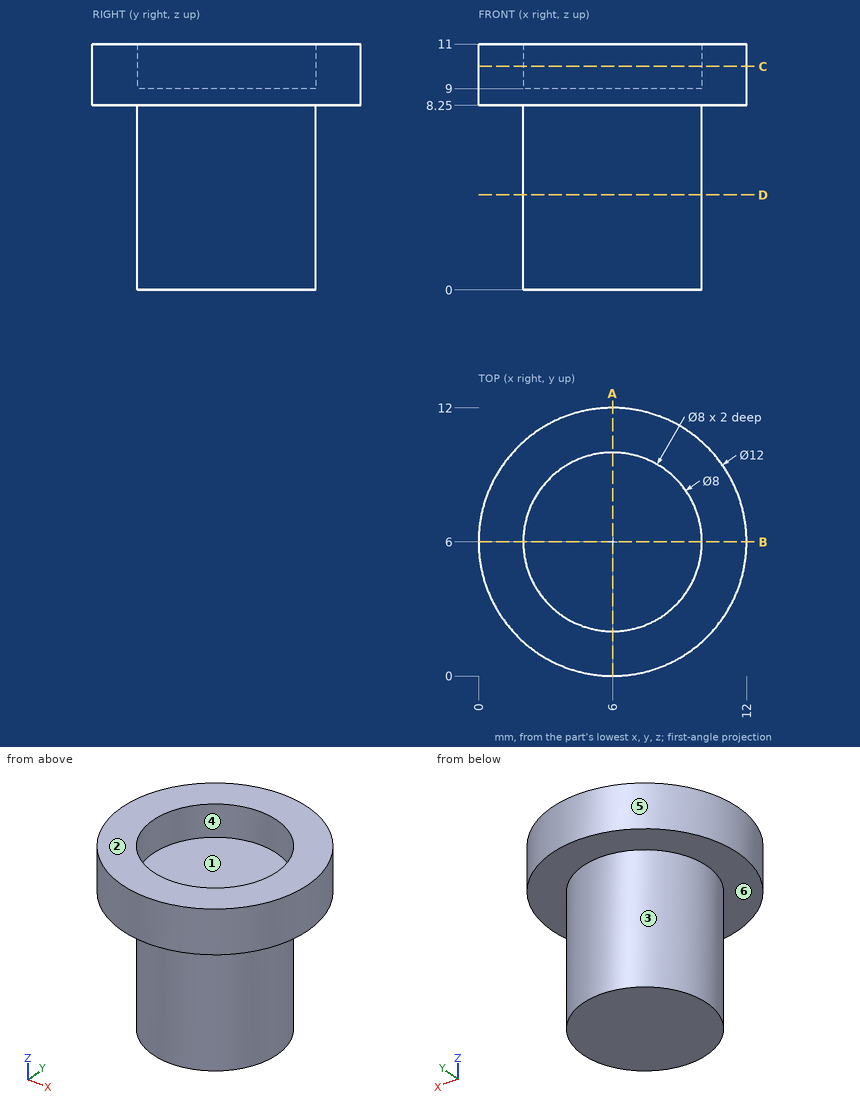
The drawing under review shows one solid part. Ordinate dimensions are in mm from its lowest x, y, z. A direction names the side the tool comes from. Coordinates: 2 decimals unless noted, no trailing zeros. Loops run counter-clockwise (first coordinate to the right, second up) from the corner with the lowest first, then second, coordinate; pieces in that order, holes last.
Item 1: Add section C-C (z = 10). Write out the cut boundary in (x, y).
Completed:
outline: circle Ø12 at (6, 6); hole circle Ø8 at (6, 6)
Item 2: Wall thickness on L1, parallel to Y at x = 6, z = 9.8; L2, parallel to Z at x = 4.25, y = 2; L3, parallel to Z at x = 3.5, y = 3: over which ranges is each line inside the solid? List them lowest first.
Completed:
L1: y = 0 to 2, 10 to 12
L2: z = 8.25 to 11
L3: z = 0 to 9
Item 3: Draft analysis for pull direction X (two halves, no side actions). For the marked faces 1, 2 and 3, state which applies: pulls with the +X half, pulls with the -X half, needs draft (parallel to the pull), parting line crosses it, or undercut.
Completed:
face 1: undercut
face 2: needs draft
face 3: parting line crosses it
Item 4: Clearance check with flat-ended pins moving along their axes: pin 1 (6.5 mm diameter, centred on x = 6, y = 6, fed in from +Z); pin 2 (3 mm diameter, centred on x = 3, z = 2, fed in from +Y); pin 3 (6 mm diameter, centred on y = 10.5, z = 7, fed in from +X). State where each tip first meets the part, or that it passes through.
Completed:
pin 1: stops at z = 9
pin 2: stops at y = 9.71
pin 3: stops at x = 11.73
Item 5: For the marked faces 4, 5 and 6, list the 3-axis set-ups (+Z, -Z, +X, -X, +Y, -Y) from which the entire face can be reached by the end or side of a thin tool; tool diameter is ignored.
Completed:
face 4: +Z
face 5: +Z, -Z
face 6: -Z
Item 6: Add section A-A (x = 6). Write out the cut boundary in (y, z), and give its area (3 significant figures).
Completed:
outline: (0, 8.25) - (2, 8.25) - (2, 0) - (10, 0) - (10, 8.25) - (12, 8.25) - (12, 11) - (10, 11) - (10, 9) - (2, 9) - (2, 11) - (0, 11) - close
area: 83.0 mm2
Item 7: Add section D-D (z = 4.25). Write out the cut boundary in (x, y).
Completed:
outline: circle Ø8 at (6, 6)
